from build123d import *

# Parameters (mm, degrees)
CROQUIS1_R              = 1.5
CROQUIS1_R_2            = 1.65
SALIENTE_EXTRUIR1_DEPTH = 2
REDONDEO1_R             = 4
CORTAR_EXTRUIR1_DEPTH   = 77.372514035
REDONDEO2_R             = 3
CROQUIS5_R              = 1.75
CORTAR_EXTRUIR2_DEPTH   = 77.372514035
CROQUIS6_R              = 2.75
CROQUIS6_R_2            = 1.75
SALIENTE_EXTRUIR6_DEPTH = 2
SALIENTE_EXTRUIR7_DEPTH = 20
CORTAR_EXTRUIR3_REACH   = 112.221
CROQUIS8_W              = 20
CROQUIS8_H              = 18
REDONDEO3_R             = 2


with BuildPart() as part:
    # Croquis1 → Saliente-Extruir1 (new body)
    with BuildSketch(Plane(origin=(0, 0, 0), x_dir=(1, 0, 0), z_dir=(0, 1, 0))):
        with BuildLine():
            Line((33.46, 41), (18.97, 54))
            Line((18.97, 54), (-41.97, 54))
            ThreePointArc((-41.97, 54), (-50.455281374, 50.485281374), (-53.97, 42))
            Line((-53.97, 42), (-53.97, -34))
            Line((-53.97, -34), (18.97, -34))
            Line((18.97, -34), (33.46, -21))
            Line((33.46, -21), (53.97, -21))
            Line((53.97, -21), (53.97, 7.59309581))
            Line((53.97, 7.59309581), (53.97, 12.40690419))
            Line((53.97, 12.40690419), (53.97, 41))
            Line((53.97, 41), (33.46, 41))
        make_face()
        with Locations(Location((-49.97, -29, 0), (0, 0, 270))):
            Circle(CROQUIS1_R, mode=Mode.SUBTRACT)
        with Locations(Location((-26.97, -10.86, 0), (0, 0, 270))):
            Circle(CROQUIS1_R_2, mode=Mode.SUBTRACT)
        with Locations(Location((14.75, -10.86, 0), (0, 0, 270))):
            Circle(CROQUIS1_R_2, mode=Mode.SUBTRACT)
        with Locations(Location((-49.97, 29, 0), (0, 0, 270))):
            Circle(CROQUIS1_R, mode=Mode.SUBTRACT)
        with Locations(Location((-26.97, 30.86, 0), (0, 0, 270))):
            Circle(CROQUIS1_R_2, mode=Mode.SUBTRACT)
        with Locations(Location((14.75, 30.86, 0), (0, 0, 270))):
            Circle(CROQUIS1_R_2, mode=Mode.SUBTRACT)
    extrude(amount=SALIENTE_EXTRUIR1_DEPTH)

    # Redondeo1
    redondeo1_edges = [part.edges().sort_by_distance(p)[0] for p in [
        (-53.97, 1, 34),
    ]]
    fillet(redondeo1_edges, radius=REDONDEO1_R)

    # Croquis4 → Cortar-Extruir1 (cut, through all)
    with BuildSketch(Plane(origin=(0, 2, 0), x_dir=(1, 0, 0), z_dir=(0, 1, 0))):
        with BuildLine():
            Line((-53.97, 26), (-53.97, -26))
            Line((-53.97, -26), (-48.47, -26))
            ThreePointArc((-48.47, -26), (-46.702233047, -25.267766953), (-45.97, -23.5))
            Line((-45.97, -23.5), (-45.97, 23.5))
            ThreePointArc((-45.97, 23.5), (-46.702233047, 25.267766953), (-48.47, 26))
            Line((-48.47, 26), (-53.97, 26))
        make_face()
    extrude(amount=-CORTAR_EXTRUIR1_DEPTH, mode=Mode.SUBTRACT)

    # Redondeo2
    redondeo2_edges = [part.edges().sort_by_distance(p)[0] for p in [
        (-53.97, 1, -26),
        (-53.97, 1, 26),
    ]]
    fillet(redondeo2_edges, radius=REDONDEO2_R)

    # Croquis5 → Cortar-Extruir2 (cut, through all)
    with BuildSketch(Plane(origin=(0, 2, 0), x_dir=(1, 0, 0), z_dir=(0, 1, 0))):
        with Locations(Location((36.97, 30, 0), (0, 0, 270))):
            Circle(CROQUIS5_R)
        with Locations(Location((36.97, -10, 0), (0, 0, 270))):
            Circle(CROQUIS5_R)
        with Locations(Location((48.97, 30, 0), (0, 0, 270))):
            Circle(CROQUIS5_R)
        with Locations(Location((48.97, -10, 0), (0, 0, 270))):
            Circle(CROQUIS5_R)
    extrude(amount=-CORTAR_EXTRUIR2_DEPTH, mode=Mode.SUBTRACT)

    # Croquis6 → Saliente-Extruir6 (add)
    # profile 1 of 4: a face of its own
    with BuildSketch(Plane.XZ):
        with Locations(Location((36.97, 10, 0), (0, 0, 270))):
            Circle(CROQUIS6_R)
        with Locations(Location((36.97, 10, 0), (0, 0, 90))):
            Circle(CROQUIS6_R_2, mode=Mode.SUBTRACT)
    # profile 2 of 4: a face of its own
    with BuildSketch(Plane.XZ):
        with Locations(Location((36.97, -30, 0), (0, 0, 270))):
            Circle(CROQUIS6_R)
        with Locations(Location((36.97, -30, 0), (0, 0, 90))):
            Circle(CROQUIS6_R_2, mode=Mode.SUBTRACT)
    # profile 3 of 4: a face of its own
    with BuildSketch(Plane.XZ):
        with Locations(Location((48.97, -30, 0), (0, 0, 270))):
            Circle(CROQUIS6_R)
        with Locations(Location((48.97, -30, 0), (0, 0, 90))):
            Circle(CROQUIS6_R_2, mode=Mode.SUBTRACT)
    # profile 4 of 4: a face of its own
    with BuildSketch(Plane.XZ):
        with Locations(Location((48.97, 10, 0), (0, 0, 270))):
            Circle(CROQUIS6_R)
        with Locations(Location((48.97, 10, 0), (0, 0, 90))):
            Circle(CROQUIS6_R_2, mode=Mode.SUBTRACT)
    extrude(amount=SALIENTE_EXTRUIR6_DEPTH)

    # Croquis7 → Saliente-Extruir7 (add)
    with BuildSketch(Plane(origin=(0, 0, 0), x_dir=(1, 0, 0), z_dir=(0, 1, 0))):
        Polygon((-41.97, -34), (18.97, -34), (33.46, -21), (34.951212399, -22.662128282), (18.97, -37), (-41.97, -37), align=None)
        Polygon((-41.97, 54), (18.97, 54), (33.46, 41), (34.951212399, 42.662128282), (18.97, 57), (-41.97, 57), align=None)
    extrude(amount=SALIENTE_EXTRUIR7_DEPTH)

    # Croquis8 → Cortar-Extruir3 (cut, up to next)
    with BuildSketch(Plane.XY.offset(37), mode=Mode.PRIVATE) as cortar_extruir3_sk1:
        with Locations((-11.03, 11)):
            Rectangle(CROQUIS8_W, CROQUIS8_H)
    cortar_extruir3_tool1 = extrude(cortar_extruir3_sk1.sketch, amount=-CORTAR_EXTRUIR3_REACH, mode=Mode.PRIVATE) & part.part
    add(cortar_extruir3_tool1.solids().sort_by_distance((-11.03, 11, 37))[0], mode=Mode.SUBTRACT)

    # Redondeo3
    # the kernel refuses this fillet: 2 mm, written as the material it adds along each edge
    with BuildSketch(Plane(origin=(-41.97, 2, 34), x_dir=(0, 0, -1), z_dir=(1, 0, 0))) as redondeo3_piece_1:
        with BuildLine():
            CenterArc((REDONDEO3_R, REDONDEO3_R), REDONDEO3_R, 180, 90)
            Line((0, REDONDEO3_R), (0, 0))
            Line((0, 0), (REDONDEO3_R, 0))
        make_face()
    extrude(amount=20.94)
    with BuildSketch(Plane(origin=(-1.03, 2, 34), x_dir=(0, 0, -1), z_dir=(1, 0, 0))) as redondeo3_piece_2_section:
        with BuildLine():
            CenterArc((REDONDEO3_R, REDONDEO3_R), REDONDEO3_R, 180, 90)
            Line((0, REDONDEO3_R), (0, 0))
            Line((0, 0), (REDONDEO3_R, 0))
        make_face()
    redondeo3_piece_2 = extrude(amount=25, mode=Mode.PRIVATE)
    redondeo3_piece_2 = split(redondeo3_piece_2, bisect_by=Plane(origin=(13.795733926, 2.442237096, 38.642198686), z_dir=(-0.6678002989650054, 0, -0.7443404870771505)), keep=Keep.TOP, mode=Mode.PRIVATE)
    add(redondeo3_piece_2)
    with BuildSketch(Plane(origin=(23.97, 2, -54), x_dir=(0, 0, 1), z_dir=(-1, 0, 0))) as redondeo3_piece_3_section:
        with BuildLine():
            CenterArc((REDONDEO3_R, REDONDEO3_R), REDONDEO3_R, 180, 90)
            Line((0, REDONDEO3_R), (0, 0))
            Line((0, 0), (REDONDEO3_R, 0))
        make_face()
    redondeo3_piece_3 = extrude(amount=65.94, mode=Mode.PRIVATE)
    redondeo3_piece_3 = split(redondeo3_piece_3, bisect_by=Plane(origin=(3.244998738, 2.450659897, -68.108006653), z_dir=(-0.6678002989650061, 0, 0.7443404870771497)), keep=Keep.TOP, mode=Mode.PRIVATE)
    add(redondeo3_piece_3)
    with BuildSketch(Plane(origin=(15.248297565, 2, 37.339001495), x_dir=(-0.6678002989650055, 0, -0.7443404870771503), z_dir=(0.7443404870771504, 0, -0.6678002989650055))) as redondeo3_piece_4_section:
        with BuildLine():
            CenterArc((REDONDEO3_R, REDONDEO3_R), REDONDEO3_R, 180, 90)
            Line((0, REDONDEO3_R), (0, 0))
            Line((0, 0), (REDONDEO3_R, 0))
        make_face()
    redondeo3_piece_4 = extrude(amount=24.466897544, mode=Mode.PRIVATE)
    redondeo3_piece_4 = split(redondeo3_piece_4, bisect_by=Plane(origin=(25.546033726, 2.446735878, 34), z_dir=(0, 0, -1)), keep=Keep.TOP, mode=Mode.PRIVATE)
    add(redondeo3_piece_4)
    with BuildSketch(Plane(origin=(33.46, 2, -41), x_dir=(-0.6678002989650058, 0, 0.74434048707715), z_dir=(-0.7443404870771501, 0, -0.6678002989650059))) as redondeo3_piece_5_section:
        with BuildLine():
            CenterArc((REDONDEO3_R, REDONDEO3_R), REDONDEO3_R, 180, 90)
            Line((0, REDONDEO3_R), (0, 0))
            Line((0, 0), (REDONDEO3_R, 0))
        make_face()
    redondeo3_piece_5 = extrude(amount=24.466897544, mode=Mode.PRIVATE)
    redondeo3_piece_5 = split(redondeo3_piece_5, bisect_by=Plane(origin=(32.635535298, 2.26154088, -54), z_dir=(0, 0, 1)), keep=Keep.TOP, mode=Mode.PRIVATE)
    add(redondeo3_piece_5)


solid = part.part
Here's how the part is built. I have some questions about the finished solid (model axes, mm). A direction names the side the tool comes from. Round coordinates to 2 decimals unless told otherwise and drop trailing zeros. Order: outer loops, then holes, each group sorted by start corner. A loop starts at its lowest first (then second) coordinate and runs counter-clockwise, first axis right, second up. Notation, with made-up numbers: M -25.75,15.25 L 13.25,15.25 A29 ccw 13.25,50.25 Z; hole C 52.25,49 d9. An arc over 180 degrees is marked long. One line per question, with ' | ' between items.
1) I'm going to push flat-ended pins straight in: pin 1 Ø12 at (x, z) = (-20, -25) entering from +Y; pin 2 Ø4 at (y, z) = (15.5, 34) entering from +X; pin 3 Ø1 at (x, y) = (-47, 1) entering from +Z; pin 4 Ø2 at (x, z) = (36.97, 10) entering from -Y. Where does each tip first touch, or does it pass through?
Checked values:
pin 1: stops at y = 2 | pin 2: stops at x = 24.54 | pin 3: stops at z = 34 | pin 4: passes through
2) I need wall thicknesses on line 1 (Z direction, x = -29, y = 8); line 2 (X direction, y = -0.7, z = -30); line 3 (X direction, y = 1.6, z = -29). Which ranges of each line are inside material? Lowest first, please.
Checked values:
line 1: z = -57 to -54, 34 to 37 | line 2: x = 34.22 to 35.22, 38.72 to 39.72, 46.22 to 47.22, 50.72 to 51.72 | line 3: x = -53.97 to -51.47, -48.47 to 35.53, 38.41 to 47.53, 50.41 to 53.97
3) Imagine slicing it at B-B, the plane y = 14.5. Write out the boundary of the cut face in (x, z), plus the area to 3 significant figures.
Checked values:
outline: M -41.97,-57 L 18.97,-57 L 34.95,-42.66 L 33.46,-41 L 18.97,-54 L -41.97,-54 Z; M -41.97,34 L -21.03,34 L -21.03,37 L -41.97,37 Z; M -1.03,34 L 18.97,34 L 33.46,21 L 34.95,22.66 L 18.97,37 L -1.03,37 Z | area: 397 mm²
4) On a 3-axis mill with a long thin cutter (end or side, diameter ignored), from which of +Z, -Z, +X, -X, +Y, -Y can I reach the whole of each face in a straight line? I mean faces 4 (the cylindrical face through (35.297, -0.986, -27.818)), 5 (the cylindrical face through (-49.9, 1, -30.5)), 6 (the cylindrical face through (-53.11, 0.99, 26.9)). Say none if no direction works.
Checked values:
face 4: -Y | face 5: +Y, -Y | face 6: -X, +Y, -Y
5) Imagine slicing it at C-C, the plane x = -9. Write out the boundary of the cut face in (y, z), plus the area to 3 significant figures.
Checked values:
outline: M 0,-57 L 20,-57 L 20,-54 L 4,-54 A2 cw 2,-52 L 2,37 L 0,37 Z | area: 243 mm²
6) Imagine slicing it at A-A, the plane x = -26.97. Write out the boundary of the cut face in (y, z).
Checked values:
outline: M 0,-57 L 20,-57 L 20,-54 L 4,-54 A2 cw 2,-52 L 2,-32.51 L 0,-32.51 Z; M 0,-29.21 L 2,-29.21 L 2,9.21 L 0,9.21 Z; M 0,12.51 L 2,12.51 L 2,32 A2 cw 4,34 L 20,34 L 20,37 L 0,37 Z
7) We'd pull the mould along X, two halves only. Please class faces 1 (the cylindrical face through (46.53, -0.99, 8.73)), 2 (the flat face through (-41.97, 10, -56)), 3 (the flat face through (37, -2, -32)): released by +X, released by -X, zero draft, split by the parting line, or undercut.
Checked values:
face 1: undercut | face 2: released by -X | face 3: zero draft
8) Imagine slicing it at D-D, the plane z = 16. Write out the boundary of the cut face in (x, y).
Checked values:
outline: M -45.97,0 L 53.97,0 L 53.97,2 L -45.97,2 Z
